Design review of the part built by this model. Coordinates are the model's own, in mm. A direction names the side the tool comes from. Coordinates: 2 decimals unless noted, no trailing zeros. Write each loop counter-clockwise with the first axis right and the second up, starting at its lowest first coordinate (ties: lowest second). Pieces come first, ordered by that corner, then holes. Notation, with made-up numbers: (-33, -17) - (9, -17) arc R15 cw to (9, -13) - close; hole circle Ø3 at (52, -16.5). An arc over 180 degrees is marked (long way). Answer as a JSON object with one key per item and string values.
```python
from build123d import *

# Parameters (mm, degrees)
EXTRUDE_1_DEPTH     = 85
EXTRUDE_2_DEPTH     = 21
CUT_EXTRUDE_1_DEPTH = 21
CUT_EXTRUDE_2_DEPTH = 21
SKETCH_4_W          = 41.549090418
SKETCH_4_H          = 35
EXTRUDE_3_DEPTH     = 21
EXTRUDE_4_DEPTH     = 21
SKETCH_7_R          = 10.5
CUT_EXTRUDE_3_DEPTH = 21


with BuildPart() as part:
    # Sketch 1 → Extrude 1 (new body)
    with BuildSketch(Plane.XY):
        with BuildLine():
            ThreePointArc((-24, 0), (-16.970562748, 16.970562748), (0, 24))
            Line((0, 24), (0, 29.218478607))
            Line((0, 29.218478607), (-28, 29.218478607))
            Line((-28, 29.218478607), (-28, 15))
            Line((-28, 15), (-77.5, 15))
            Line((-77.5, 15), (-77.5, 0))
            Line((-77.5, 0), (-24, 0))
        make_face()
        with BuildLine():
            Line((0, 29.218478607), (0, 24))
            ThreePointArc((0, 24), (16.970562748, 16.970562748), (24, 0))
            Line((24, 0), (77.5, 0))
            Line((77.5, 0), (77.5, 15))
            Line((77.5, 15), (28, 15))
            Line((28, 15), (28, 29.218478607))
            Line((28, 29.218478607), (0, 29.218478607))
        make_face()
    extrude(amount=EXTRUDE_1_DEPTH)

    # Sketch 1_3 → Extrude 2 (add)
    with BuildSketch(Plane.XY):
        Polygon((-28, 29.218478607), (0, 29.218478607), (0, 57), (-20.774545209, 57), (-20.774545209, 78), (-77.5, 15), (-28, 15), align=None)
        Polygon((0, 57), (0, 29.218478607), (28, 29.218478607), (28, 15), (77.5, 15), (20.774545209, 78), (20.774545209, 57), align=None)
    extrude(amount=EXTRUDE_2_DEPTH)

    # Sketch 3 → Cut-Extrude 1 (cut)
    with BuildSketch(Plane(origin=(0, 15, 0), x_dir=(1, 0, 0), z_dir=(0, 1, 0))):
        with BuildLine():
            ThreePointArc((77.5, -67), (72.227922061, -79.727922061), (59.5, -85))
            Line((59.5, -85), (77.5, -85))
            Line((77.5, -85), (77.5, -67))
        make_face()
    extrude(amount=-CUT_EXTRUDE_1_DEPTH, mode=Mode.SUBTRACT)

    # Sketch 2 → Cut-Extrude 2 (cut)
    with BuildSketch(Plane(origin=(0, 15, 0), x_dir=(1, 0, 0), z_dir=(0, 1, 0))):
        with BuildLine():
            ThreePointArc((-59.5, -85), (-72.227922061, -79.727922061), (-77.5, -67))
            Line((-77.5, -67), (-77.5, -85))
            Line((-77.5, -85), (-59.5, -85))
        make_face()
    extrude(amount=-CUT_EXTRUDE_2_DEPTH, mode=Mode.SUBTRACT)

    # Sketch 4 → Extrude 3 (add)
    with BuildSketch(Plane(origin=(0, 57, 0), x_dir=(1, 0, 0), z_dir=(0, 1, 0))):
        with Locations((0, -17.5)):
            Rectangle(SKETCH_4_W, SKETCH_4_H)
    extrude(amount=EXTRUDE_3_DEPTH)

    # Sketch 5 → Extrude 4 (add)
    with BuildSketch(Plane(origin=(0, 78, 0), x_dir=(1, 0, 0), z_dir=(0, 1, 0))):
        with BuildLine():
            Line((10.5, -35), (20.774545209, -35))
            ThreePointArc((20.774545209, -35), (0, -14.225454791), (-20.774545209, -35))
            Line((-20.774545209, -35), (-10.5, -35))
            ThreePointArc((-10.5, -35), (0, -24.5), (10.5, -35))
        make_face()
        with BuildLine():
            ThreePointArc((-20.774545209, -35), (0, -55.774545209), (20.774545209, -35))
            Line((20.774545209, -35), (10.5, -35))
            ThreePointArc((10.5, -35), (0, -45.5), (-10.5, -35))
            Line((-10.5, -35), (-20.774545209, -35))
        make_face()
    extrude(amount=-EXTRUDE_4_DEPTH)

    # Sketch 7 → Cut-Extrude 3 (cut)
    with BuildSketch(Plane(origin=(0, 78, 0), x_dir=(1, 0, 0), z_dir=(0, 1, 0))):
        with Locations(Location((0, -35, 0), (0, 0, 270))):
            Circle(SKETCH_7_R)
    extrude(amount=-CUT_EXTRUDE_3_DEPTH, mode=Mode.SUBTRACT)


solid = part.part
```
(1) Take a section at C-C, the plane x = -6.5. Write out the cut boundary in (y, z), and give its area (3 significant figures).
Solved:
{"outline": "(23.1, 0) - (78, 0) - (78, 26.75) - (57, 26.75) - (57, 21) - (29.22, 21) - (29.22, 85) - (23.1, 85) - close; (57, 43.25) - (78, 43.25) - (78, 54.73) - (57, 54.73) - close", "area": "1,910 mm^2"}
(2) Tool access review of faces 5 (the face through (-28, 22, 53)), 6 (the face through (0, 57, 46)), 7 (the face through (53, 15, 53)): name each direction out of +Z, -Z, +X, -X, +Y, -Y from which nothing blocks a thin tool from reaching the whole face with its end or side.
Solved:
{"face 5": "+Z, -X, +Y", "face 6": "+Z, +X, -X", "face 7": "+Z, +X, +Y"}
(3) Take a section at D-D, the plane z = 62. Write out the cut boundary in (x, y).
Solved:
{"outline": "(-77.5, 0) - (-24, 0) arc R24 cw to (24, 0) - (77.5, 0) - (77.5, 15) - (28, 15) - (28, 29.22) - (-28, 29.22) - (-28, 15) - (-77.5, 15) - close"}
(4) To check wall thickness, follow line 1 (X direction, y = 63, z = 35); line 2 (Y direction, x = 55.5, z = 29); line 3 (Z direction, x = -24, y = 31.5). State the ranges of each line that lie inside material, in increasing order. Write a range as from..to.
Solved:
{"line 1": "x = -20.77..-10.5, 10.5..20.77", "line 2": "y = 0..15", "line 3": "z = 0..21"}
(5) Take a section at A-A, the plane y = 6. Write out the cut boundary in (x, z), and give its area (3 significant figures).
Solved:
{"outline": "(-77.5, 0) - (-23.24, 0) - (-23.24, 85) - (-59.5, 85) arc R18 ccw to (-77.5, 67) - close; (23.24, 0) - (77.5, 0) - (77.5, 67) arc R18 ccw to (59.5, 85) - (23.24, 85) - close", "area": "9,090 mm^2"}
(6) Take a section at B-B, the plane z = 39.5. Write out the cut boundary in (x, y), and give its area (3 significant figures).
Solved:
{"outline": "(-77.5, 0) - (-24, 0) arc R24 cw to (24, 0) - (77.5, 0) - (77.5, 15) - (28, 15) - (28, 29.22) - (-28, 29.22) - (-28, 15) - (-77.5, 15) - close; (-20.28, 57) - (-9.49, 57) - (-9.49, 78) - (-20.28, 78) - close; (9.49, 57) - (20.28, 57) - (20.28, 78) - (9.49, 78) - close", "area": "2,670 mm^2"}
(7) The part is to be moulded in two halves that separate along X. For faces 1 (the face through (-72.087, 7.605, 79.867)), 2 (the face through (0.46, 67.65, 24.51)), 3 (the face through (72.367, 7.605, 79.587)), 4 (the face through (-0.46, 67.65, 55.77)), say which applies: pulls with the +X half, pulls with the -X half, needs draft (parallel to the pull), parting line crosses it, or undercut.
Solved:
{"face 1": "pulls with the -X half", "face 2": "undercut", "face 3": "pulls with the +X half", "face 4": "parting line crosses it"}
(8) For pin 1 (2 mm diameter, centred on y = 70, z = 44, fed in from +X); pin 2 (19 mm diameter, centred on x = 0, z = 35, fed in from -Y); pin 3 (12 mm diameter, centred on x = -22, y = 63.5, fed in from +Z), all flat-tipped, find the tip position at first contact; note any pin that passes through.
Solved:
{"pin 1": "stops at x = 19.17", "pin 2": "stops at y = 22.04", "pin 3": "stops at z = 48.25"}
